The listing builds one solid part. Answer for the finished solid, in the listing's coordinates (mm). A direction names the side the tool comes from. Give positions to 0.01 mm unless a question says otherwise; leave off trailing zeros. Loops run counter-clockwise (first coordinate to the right, second up) from the corner with the lowest first, then second, coordinate; pieces in that order, holes last.
Item 1: The mould has two halves that part along X. Classify faces 3 (the face through (-14.57, -3.13, 33.85)), 4 (the face through (9, 0, 9)): pulls with the +X half, pulls with the -X half, needs draft (parallel to the pull), parting line crosses it, or undercut.
Item 2: Section A-A, the plane x = 0 is taken. Give the vertices of the cut face in (y, z) (3 decimals).
Item 3: A tool of negligible diameter and unlimited length cuts with its end or side. For faces 1 (the face through (13.58, -3.13, 15.45)), 2 (the face through (9, -6.35, 9)), from which of +Z, -Z, +X, -X, +Y, -Y can it reach the whole face along a straight path? Write none if from no direction.
Item 4: Consider line 1 along Z through (x, y) = (0, -2.75) (3 decimals); line 2 along X through (y, z) = (-5.75, 6); line 3 along X through (y, z) = (-1.75, -20). Determine where each line is inside the solid, lowest interval first.
Item 5: This flat-tipped pin is pushed along its axis until it touches: pin 1 Ø2 at (y, z) = (-2.5, 12.5) entering from +X. Where does it stop, or does it pass through?
Item 6: Section C-C, the plane y = -5.25 is taken. Give the number of separate pieces and of enclosed holes in the cut face, and give its area (3 significant figures).
Item 7: Section B-B, the plane x = 29 is taken. Give the vertices of the cut face in (y, z).
Item 8: Section D-D, the plane x = -37.5 is taken. Give the vertices of the cut face in (y, z).
from build123d import *

# Parameters (mm, degrees)
F0_R     = 11.2395
F1_DEPTH = 6.35


# Not quite as in the source:
# - ends of sketch curves that miss each other by under 0.0002 mm in the source are joined


with BuildPart() as f1:
    # F0 (on Front) → F1 (new body)
    with BuildSketch(Plane.XZ):
        with BuildLine():
            Line((42.4466417494, 1.2702137502), (33.5675281941, 16.6492895541))
            Line((33.5675281941, 16.6492895541), (21.59, 37.3949769354))
            Line((21.59, 37.3949769354), (-2.3645964913, 37.3949769354))
            Line((-2.3645964913, 37.3949769354), (-20.1530883691, 37.3949769354))
            ThreePointArc((-20.1530883691, 37.3949769354), (-21.3957267903, 37.0536052726), (-22.3109030797, 36.1463361741))
            Line((-22.3109030797, 36.1463361741), (-31.2024712814, 20.7456882897))
            Line((-31.2024712814, 20.7456882897), (-43.18, 0))
            Line((-43.18, 0), (-31.2026751276, -20.7453352178))
            Line((-31.2026751276, -20.7453352178), (-22.3013335195, -36.1629111385))
            ThreePointArc((-22.3013335195, -36.1629111385), (-21.904358157, -36.6666327955), (-21.3938662061, -37.0548632868))
            ThreePointArc((-21.3938662061, -37.0548632868), (-20.7960911396, -37.3045921602), (-20.1545849957, -37.3949769354))
            Line((-20.1545849957, -37.3949769354), (-2.3645964913, -37.3949769354))
            Line((-2.3645964913, -37.3949769354), (21.59, -37.3949769354))
            Line((21.59, -37.3949769354), (33.5675281941, -16.6492895541))
            Line((33.5675281941, -16.6492895541), (42.4465800457, -1.269893127))
            Line((42.4465800457, -1.269893127), (42.4466570355, -1.2697597731))
            ThreePointArc((42.4466570355, -1.2697597731), (42.7869372237, 0.0002290365), (42.4466417494, 1.2702137502))
        make_face()
        with Locations((-13.1097560234, -22.7067635073)):
            Circle(F0_R, mode=Mode.SUBTRACT)
        Polygon((19.322999251, -17.547366104), (14.6677320258, -25.4052571005), (5.5348901331, -25.5078921242), (7.6610986638, -13.3857599047), (7.676716044, -13.2967206855), align=None, mode=Mode.SUBTRACT)
        Polygon((-15.3534299541, -0.0001902285), (-24.8221534826, -7.8882218978), (-24.8579644411, -7.9605251767), (-29.3354640516, 0), (-24.8579276431, 7.9605905996), (-24.8220816566, 7.8883561733), (-17.7474034479, 1.9942828585), align=None, mode=Mode.SUBTRACT)
        with Locations((-13.1097560234, 22.7067635073)):
            Circle(F0_R, mode=Mode.SUBTRACT)
        with BuildLine():
            ThreePointArc((-4.7625, 8.248891971), (4.7625, 8.248891971), (9.525, 0))
            ThreePointArc((9.525, 0), (-4.7625, -8.248891971), (-4.7625, 8.248891971))
        make_face(mode=Mode.SUBTRACT)
        with Locations((26.2195120463, 0.0001612286)):
            Circle(F0_R, mode=Mode.SUBTRACT)
        Polygon((5.5348901331, 25.5078921242), (14.6677320258, 25.4052571005), (19.322999251, 17.547366104), (7.676716044, 13.2967206855), (7.6610986638, 13.3857599047), align=None, mode=Mode.SUBTRACT)
        with BuildLine():
            Line((43.18, 0), (42.4466417494, 1.2702137502))
            ThreePointArc((42.4466417494, 1.2702137502), (42.7869372237, 0.0002290365), (42.4466570355, -1.2697597731))
            Line((42.4466570355, -1.2697597731), (42.4465800457, -1.269893127))
            Line((42.4465800457, -1.269893127), (33.5675281941, -16.6492895541))
            Line((33.5675281941, -16.6492895541), (43.18, 0))
        make_face()
        with BuildLine():
            Line((-20.1530883691, 37.3949769354), (-2.3645964913, 37.3949769354))
            Line((-2.3645964913, 37.3949769354), (-20.1235435545, 37.3951484857))
            ThreePointArc((-20.1235435545, 37.3951484857), (-20.1383162113, 37.3951056691), (-20.1530883691, 37.3949769354))
        make_face()
        with BuildLine():
            ThreePointArc((-22.3109030797, 36.1463361741), (-21.3957267903, 37.0536052726), (-20.1530883691, 37.3949769354))
            Line((-20.1530883691, 37.3949769354), (-21.59, 37.3949769354))
            Line((-21.59, 37.3949769354), (-22.3109030797, 36.1463361741))
        make_face()
        with BuildLine():
            Line((-31.2024712814, 20.7456882897), (-22.3109030797, 36.1463361741))
            ThreePointArc((-22.3109030797, 36.1463361741), (-22.3171177275, 36.1357499036), (-22.3232811402, 36.125133722))
            Line((-22.3232811402, 36.125133722), (-31.2024712814, 20.7456882897))
        make_face()
        with BuildLine():
            Line((-20.1238326592, -37.395162783), (-2.3645964913, -37.3949769354))
            Line((-2.3645964913, -37.3949769354), (-20.1545849957, -37.3949769354))
            ThreePointArc((-20.1545849957, -37.3949769354), (-20.1392091087, -37.3951164012), (-20.1238326592, -37.395162783))
        make_face()
        with BuildLine():
            Line((-21.59, -37.3949769354), (-20.1545849957, -37.3949769354))
            ThreePointArc((-20.1545849957, -37.3949769354), (-20.7960911396, -37.3045921602), (-21.3938662061, -37.0548632868))
            Line((-21.3938662061, -37.0548632868), (-21.590116174, -37.3947757161))
            Line((-21.590116174, -37.3947757161), (-21.59, -37.3949769354))
        make_face()
        with BuildLine():
            Line((-21.590116174, -37.3947757161), (-21.3938662061, -37.0548632868))
            ThreePointArc((-21.3938662061, -37.0548632868), (-21.904358157, -36.6666327955), (-22.3013335195, -36.1629111385))
            Line((-22.3013335195, -36.1629111385), (-21.590116174, -37.3947757161))
        make_face()
        with BuildLine():
            Line((-22.3013335195, -36.1629111385), (-31.2026751276, -20.7453352178))
            Line((-31.2026751276, -20.7453352178), (-22.3235850993, -36.1251258309))
            ThreePointArc((-22.3235850993, -36.1251258309), (-22.3125408514, -36.1440665044), (-22.3013335195, -36.1629111385))
        make_face()
    extrude(amount=F1_DEPTH)


solid = f1.part
Worked answers:
1. face 3: undercut
1. face 4: needs draft
2. outline: (-6.35, -37.395) - (0, -37.395) - (0, -9.525) - (-6.35, -9.525) - close; (-6.35, 9.525) - (0, 9.525) - (0, 37.395) - (-6.35, 37.395) - close
3. face 1: +Y, -Y
3. face 2: +Z, -Z, +X, -X, -Y
4. line 1: z = -37.395 to -9.525, 9.525 to 37.395
4. line 2: x = -39.72 to -25.96, -22.56 to -7.4, 7.4 to 16.72, 35.72 to 39.72
4. line 3: x = -31.63 to -24.02, -2.2 to 6.5, 17.87 to 31.63
5. pin 1: stops at x = 36.54
6. separate pieces: 1
6. enclosed holes: 7
6. area: 3,040 mm2
7. outline: (-6.35, -24.56) - (0, -24.56) - (0, -10.89) - (-6.35, -10.89) - close; (-6.35, 10.89) - (0, 10.89) - (0, 24.56) - (-6.35, 24.56) - close
8. outline: (-6.35, -9.84) - (0, -9.84) - (0, 9.84) - (-6.35, 9.84) - close
